```python
from build123d import *

# Parameters (mm, degrees)
SKETCH_1_W               = 28
SKETCH_1_H               = 55
SKETCH_1_R               = 1.5
EXTRUDE_1_DEPTH          = 5
CUT_EXTRUDE_1_DEPTH      = 62.919302322
CUT_EXTRUDE_1_DEPTH_BACK = 4
SKETCH_4_R               = 0.85
SKETCH_5_W               = 55
SKETCH_5_H               = 5
EXTRUDE_2_DEPTH          = 5
SKETCH_1_22_R            = 1.5
CUT_EXTRUDE_2_DEPTH      = 62.919302322
SKETCH_1_23_R            = 2.25
CUT_EXTRUDE_3_DEPTH      = 3


with BuildPart() as part:
    # 草图1 → 凸台-拉伸1 (new body)
    with BuildSketch(Plane(origin=(0, 0, 0), x_dir=(1, 0, 0), z_dir=(0, 1, 0))):
        with Locations((-14, -27.5)):
            Rectangle(SKETCH_1_W, SKETCH_1_H)
        with Locations(Location((-23, -24.5, 0), (0, 0, 270))):
            Circle(SKETCH_1_R, mode=Mode.SUBTRACT)
        with Locations(Location((-5, -24.5, 0), (0, 0, 270))):
            Circle(SKETCH_1_R, mode=Mode.SUBTRACT)
        with Locations(Location((-13, -52.5, 0), (0, 0, 270))):
            Circle(SKETCH_1_R, mode=Mode.SUBTRACT)
        with Locations(Location((-23, -52.5, 0), (0, 0, 270))):
            Circle(SKETCH_1_R, mode=Mode.SUBTRACT)
    extrude(amount=EXTRUDE_1_DEPTH)

    # 草图4 → 切除-拉伸1 (cut, two sides: drawn at the far end of the back side and taken through both)
    with BuildSketch(Plane.ZY.offset(28).offset(-CUT_EXTRUDE_1_DEPTH_BACK)):
        with Locations(Location((10, 2.5, 0), (0, 0, 180))):
            Circle(SKETCH_4_R)
        with Locations(Location((45, 2.5, 0), (0, 0, 180))):
            Circle(SKETCH_4_R)
    extrude(amount=CUT_EXTRUDE_1_DEPTH + CUT_EXTRUDE_1_DEPTH_BACK, mode=Mode.SUBTRACT)

    # 草图5 → 凸台-拉伸2 (add)
    with BuildSketch(Plane(origin=(0, 0, 0), x_dir=(0, 0, -1), z_dir=(1, 0, 0))):
        with Locations((-27.5, 2.5)):
            Rectangle(SKETCH_5_W, SKETCH_5_H)
    extrude(amount=EXTRUDE_2_DEPTH)

    # 草图1<22> → 切除-拉伸2 (cut, through all)
    with BuildSketch(Plane(origin=(0, 0, 0), x_dir=(1, 0, 0), z_dir=(0, 1, 0))):
        with Locations(Location((2.5, -37.701964887, 0), (0, 0, 270))):
            Circle(SKETCH_1_22_R)
        with Locations(Location((2.5, -10, 0), (0, 0, 270))):
            Circle(SKETCH_1_22_R)
    extrude(amount=CUT_EXTRUDE_2_DEPTH, mode=Mode.SUBTRACT)

    # 草图1<23> → 切除-拉伸3 (cut)
    with BuildSketch(Plane(origin=(0, 0, 0), x_dir=(1, 0, 0), z_dir=(0, 1, 0))):
        with Locations(Location((-23, -24.5, 0), (0, 0, 270))):
            Circle(SKETCH_1_23_R)
        with Locations(Location((-5, -24.5, 0), (0, 0, 270))):
            Circle(SKETCH_1_23_R)
        with Locations(Location((-13, -52.5, 0), (0, 0, 270))):
            Circle(SKETCH_1_23_R)
        with Locations(Location((2.5, -37.701964887, 0), (0, 0, 270))):
            Circle(SKETCH_1_23_R)
        with Locations(Location((-23, -52.5, 0), (0, 0, 270))):
            Circle(SKETCH_1_23_R)
        with Locations(Location((2.5, -10, 0), (0, 0, 270))):
            Circle(SKETCH_1_23_R)
    extrude(amount=CUT_EXTRUDE_3_DEPTH, mode=Mode.SUBTRACT)


solid = part.part
```
The model under review builds one solid part; all positions refer to its coordinate system, in mm. A direction names the side the tool comes from. Round coordinates to 2 decimals unless told otherwise and drop trailing zeros. Loops run counter-clockwise (first coordinate to the right, second up) from the corner with the lowest first, then second, coordinate; pieces in that order, holes last. Notation, with made-up numbers: M 67.5,-22.75 L 83.5,-22.75 A12 cw 83.5,-10.75 Z; hole C -1,18 d10. An arc over 180 degrees is marked long. Answer as a JSON object with one key per item and string values.
(1) Take a section at A-A on x = 2.5. Give the boundary of the cut face in (y, z), and give its area (3 significant figures).
Resolved:
{"outline": "M 0,0 L 5,0 L 5,8.5 L 3,8.5 L 3,7.75 L 0,7.75 Z; M 0,12.25 L 3,12.25 L 3,11.5 L 5,11.5 L 5,36.2 L 3,36.2 L 3,35.45 L 0,35.45 Z; M 0,39.95 L 3,39.95 L 3,39.2 L 5,39.2 L 5,55 L 0,55 Z", "area": "236 mm²"}
(2) Tool access review of faces 3 (the cylindrical face through (-24.996, 1.479, 25.538)), 4 (the cylindrical face through (-25.972, 2.826, 9.215)), 5 (the cylindrical face through (-13.9, 4, 51.3)): name each direction out of +Z, -Z, +X, -X, +Y, -Y from which nothing blocks a thin tool from reaching the whole face with its end or side.
Resolved:
{"face 3": "-Y", "face 4": "-X", "face 5": "+Y, -Y"}
(3) To check wall thickness, follow line 1 along X through (y, z) = (1.7, 24.5); line 2 along Z through (x, y) = (-23, 3.45); line 3 along X through (y, z) = (3.7, 52.5). State the ranges of each line that lie inside material, in increasing order.
Resolved:
{"line 1": "-28 to -25.25, -20.75 to -7.25, -2.75 to 5", "line 2": "0 to 23, 26 to 51, 54 to 55", "line 3": "-28 to -24.5, -21.5 to -14.5, -11.5 to 5"}
(4) Take a section at C-C on x = -13. Give the boundary of the cut face in (y, z).
Resolved:
{"outline": "M 0,0 L 5,0 L 5,51 L 3,51 L 3,50.25 L 0,50.25 Z; M 0,54.75 L 3,54.75 L 3,54 L 5,54 L 5,55 L 0,55 Z"}
(5) Take a section at D-D on y = 4. Give the boundary of the cut face in (x, z), and give its area (3 significant figures).
Resolved:
{"outline": "M -28,0 L 5,0 L 5,55 L -28,55 Z; hole C -23,24.5 d3; hole C -23,52.5 d3; hole C -13,52.5 d3; hole C -5,24.5 d3; hole C 2.5,10 d3; hole C 2.5,37.7 d3", "area": "1,770 mm²"}
(6) Draft analysis for pull direction Z (two halves, no side actions). For faces 1 (the flat face through (1, 3, 9)), 2 (the flat face through (5, 3, 28)), state which applies: released by +Z, released by -Z, zero draft, split by the parting line, or undercut.
Resolved:
{"face 1": "undercut", "face 2": "zero draft"}
(7) Take a section at B-B on z = 52.5. Give the boundary of the cut face in (x, y).
Resolved:
{"outline": "M -28,0 L -25.25,0 L -25.25,3 L -24.5,3 L -24.5,5 L -28,5 Z; M -21.5,3 L -20.75,3 L -20.75,0 L -15.25,0 L -15.25,3 L -14.5,3 L -14.5,5 L -21.5,5 Z; M -11.5,3 L -10.75,3 L -10.75,0 L 5,0 L 5,5 L -11.5,5 Z"}
(8) Clearance check with flat-ended pins moving along their axes: P1, Ø1.3, axis at x = -13, z = 53.5, coming from the -Y side; P2, Ø2.5, axis at x = 2.5, z = 10, coming from the +Y side. State where each tip first meets the part, or that it passes through.
Resolved:
{"P1": "y = 3", "P2": "through"}
